from build123d import *

# Parameters (mm, degrees)
F0_R     = 9.756
F1_DEPTH = 25.4


with BuildPart() as f1:
    # F0 (on Right) → F1 (new body)
    with BuildSketch(Plane.YZ):
        with Locations((-0.415131, 0.719028)):
            Circle(F0_R)
        Polygon((6.226969, 4.553847), (6.226969, -3.11579), (-0.415131, -6.950608), (-7.057231, -3.11579), (-7.057231, 4.553847), (-0.415131, 8.388665), align=None, mode=Mode.SUBTRACT)
    extrude(amount=F1_DEPTH)


solid = f1.part
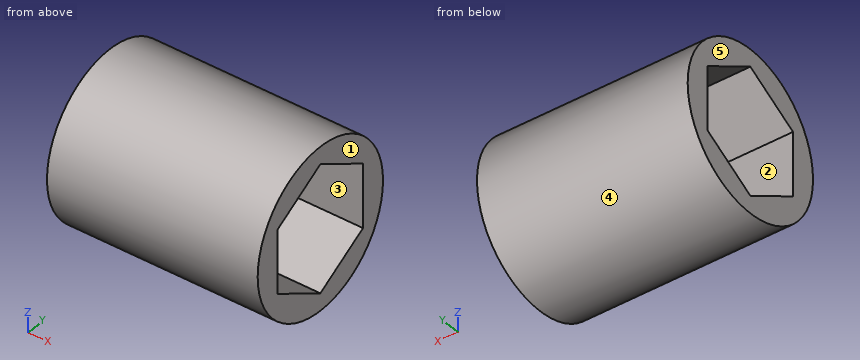
Verification items for the finished model (mm, model axes). Face numbers are marked on the shaded views. A direction names the side the tool comes from. Coordinates: 2 decimals unless noted, no trailing zeros. Order: outer loops, then holes, each group sorted by start corner. A loop starts at its lowest first (then second) coordinate and runs counter-clockwise, first axis right, second up. Notation, with made-up numbers: (17, 37) -> (48, 37) arc R21 ccw to (48, 51) -> close; hole circle Ø10 at (58, 89). An arc over 180 degrees is marked (long way). Put each result on its own line as item: value. Start each with the question number.
1. Mould release check, pull along Y, two halves, no side actions. Record for the marked faces 3, 4 and 5: released by +Y, released by -Y, zero draft, split by the parting line, or undercut.
2. Access from +Z, -Z, +X, -X, +Y, -Y to the whole of each face (thin tool, end or side, straight path). Record for the marked faces 1 and 2.
3. Cross-section at A-A, the plane z = 3. Record the boundary of the cut face in (x, y), then the cut area to 3 significant figures.
4. Cross-section at B-B, the plane y = -3.25. Record the boundary of the cut face in (x, z).
5. Go/stop test with flat-tipped pins: pin 1 Ø4 at (x, z) = (5, -4.5) entering from +Y; pin 2 Ø8 at (x, z) = (12, -6) entering from -Y; pin 3 Ø10 at (x, y) = (10.5, -6) entering from -Z. Record where each tip stops, or that it passes through.
6. Cross-section at D-D, the plane y = -8. Record the boundary of the cut face in (x, z), then the cut area to 3 significant figures.
7. Cross-section at C-C, the plane x = 23.5. Record the boundary of the cut face in (y, z), then the cut area to 3 significant figures.
8. Material ranges on L1, parallel to Y at x = 10.25, z = 5.25; L2, parallel to Z at x = 16.75, y = 4.75; L3, parallel to Y at x = 1.75, z = -2.75, recorded low to high. Write a range as [from, to].
Computed:
1. face 3: undercut
1. face 4: split by the parting line
1. face 5: zero draft
2. face 1: +Z, -Z, +X, +Y, -Y
2. face 2: +X, -X
3. outline: (0, -9.9) -> (25.4, -9.9) -> (25.4, -7.06) -> (0, -7.06) -> close; (0, 6.23) -> (25.4, 6.23) -> (25.4, 9.07) -> (0, 9.07) -> close
3. area: 144 mm2
4. outline: (0, -8.62) -> (25.4, -8.62) -> (25.4, -5.31) -> (0, -5.31) -> close; (0, 6.75) -> (25.4, 6.75) -> (25.4, 10.05) -> (0, 10.05) -> close
5. pin 1: y = 8.79
5. pin 2: y = -9.78
5. pin 3: z = -9.02
6. outline: (0, -5.42) -> (25.4, -5.42) -> (25.4, 6.85) -> (0, 6.85) -> close
6. area: 312 mm2
7. outline: circle Ø19.51 at (-0.42, 0.72); hole (-7.06, -3.12) -> (-0.42, -6.95) -> (6.23, -3.12) -> (6.23, 4.55) -> (-0.42, 8.39) -> (-7.06, 4.55) -> close
7. area: 146 mm2
8. L1: [-9.06, -5.85], [5.02, 8.22]
8. L2: [-7.56, -3.97], [5.41, 9]
8. L3: [-9.53, -7.06], [6.23, 8.7]
